For this review, take the finished solid that the model builds, in its own axes (mm). Face numbers are marked on the shaded views. A direction names the side the tool comes from. Give positions to 0.01 mm unless a question says otherwise; leave off trailing zeros. Order: outer loops, then holes, each group sorted by start corner. A loop starts at its lowest first (then second) coordinate and runs counter-clockwise, first axis right, second up. Notation, with made-up numbers: (21.25, 84) - (62.25, 84) arc R5 cw to (62.25, 90) - close; hole circle Ø5 at (21.5, 60.25). An arc over 180 degrees is marked (long way). Put each result on its own line as item: value. Start each with the question number.
```python
from build123d import *

# Parameters (mm, degrees)
SKETCH2_W                                           = 25
SKETCH2_H                                           = 25
BOSS_EXTRUDE1_DEPTH                                 = 10
SKETCH3_W                                           = 20
SKETCH3_H                                           = 20
CUT_EXTRUDE1_DEPTH                                  = 21.310096012
SKETCH5_W                                           = 10
SKETCH5_H                                           = 20
BOSS_EXTRUDE2_DEPTH                                 = 15
SKETCH7_W                                           = 12
SKETCH7_H                                           = 10
CUT_EXTRUDE2_DEPTH                                  = 40.477841886
SKETCH8_R                                           = 2.25
CUT_EXTRUDE3_DEPTH                                  = 49.757050772
SKETCH9_R                                           = 1.75
CUT_EXTRUDE4_DEPTH                                  = 15
SKETCH10_R                                          = 1.75
CUT_EXTRUDE5_DEPTH                                  = 15
CBORE_FOR_M4_HEX_SOCKET_HEAD_CAP_SCREW1_D           = 4.5
CBORE_FOR_M4_HEX_SOCKET_HEAD_CAP_SCREW1_CBORE_D     = 8
CBORE_FOR_M4_HEX_SOCKET_HEAD_CAP_SCREW1_CBORE_DEPTH = 3
CUT_EXTRUDE6_DEPTH                                  = 3


with BuildPart() as part:
    # Sketch2 → Boss-Extrude1 (new body)
    with BuildSketch(Plane.XY):
        Rectangle(SKETCH2_W, SKETCH2_H)
    extrude(amount=BOSS_EXTRUDE1_DEPTH)

    # Sketch3 → Cut-Extrude1 (cut, through all)
    with BuildSketch(Plane.XY.offset(10)):
        with Locations((-2.5, -2.5)):
            Rectangle(SKETCH3_W, SKETCH3_H)
    extrude(amount=-CUT_EXTRUDE1_DEPTH, mode=Mode.SUBTRACT)

    # Sketch5 → Boss-Extrude2 (add)
    with BuildSketch(Plane(origin=(12.5, 0, 0), x_dir=(0, 0, -1), z_dir=(1, 0, 0))):
        with Locations((-5, 16.5)):
            Rectangle(SKETCH5_W, SKETCH5_H)
    extrude(amount=BOSS_EXTRUDE2_DEPTH)

    # Sketch7 → Cut-Extrude2 (cut, through all)
    with BuildSketch(Plane.XY.offset(10)):
        with Locations((21.5, 16.5)):
            Rectangle(SKETCH7_W, SKETCH7_H)
    extrude(amount=-CUT_EXTRUDE2_DEPTH, mode=Mode.SUBTRACT)

    # Sketch8 → Cut-Extrude3 (cut, through all)
    with BuildSketch(Plane(origin=(0, 26.5, 0), x_dir=(1, 0, 0), z_dir=(0, 1, 0))):
        with Locations(Location((22.5, -5, 0), (0, 0, 270))):
            Circle(SKETCH8_R)
    extrude(amount=-CUT_EXTRUDE3_DEPTH, mode=Mode.SUBTRACT)

    # Sketch9 → Cut-Extrude4 (cut)
    with BuildSketch(Plane(origin=(0, 12.5, 0), x_dir=(1, 0, 0), z_dir=(0, 1, 0))):
        with Locations(Location((-2.5, -5, 0), (0, 0, 270))):
            Circle(SKETCH9_R)
    extrude(amount=-CUT_EXTRUDE4_DEPTH, mode=Mode.SUBTRACT)

    # Sketch10 → Cut-Extrude5 (cut)
    with BuildSketch(Plane(origin=(12.5, 0, 0), x_dir=(0, 0, -1), z_dir=(1, 0, 0))):
        with Locations((-5, -2.5)):
            Circle(SKETCH10_R)
    extrude(amount=-CUT_EXTRUDE5_DEPTH, mode=Mode.SUBTRACT)

    # CBORE for M4 Hex Socket Head Cap Screw1 (through all)
    with Locations(Plane(origin=(0, 26.5, 0), x_dir=(1, 0, 0), z_dir=(0, 1, 0))):
        with Locations((22.5, -5)):
            CounterBoreHole(CBORE_FOR_M4_HEX_SOCKET_HEAD_CAP_SCREW1_D / 2, CBORE_FOR_M4_HEX_SOCKET_HEAD_CAP_SCREW1_CBORE_D / 2, CBORE_FOR_M4_HEX_SOCKET_HEAD_CAP_SCREW1_CBORE_DEPTH)

    # Sketch13 → Cut-Extrude6 (cut)
    with BuildSketch(Plane.XZ.offset(-6.5)):
        Polygon((17.881197846, 5), (20.190598923, 1), (24.809401077, 1), (27.118802154, 5), (24.809401077, 9), (20.190598923, 9), align=None)
    extrude(amount=-CUT_EXTRUDE6_DEPTH, mode=Mode.SUBTRACT)


solid = part.part
```
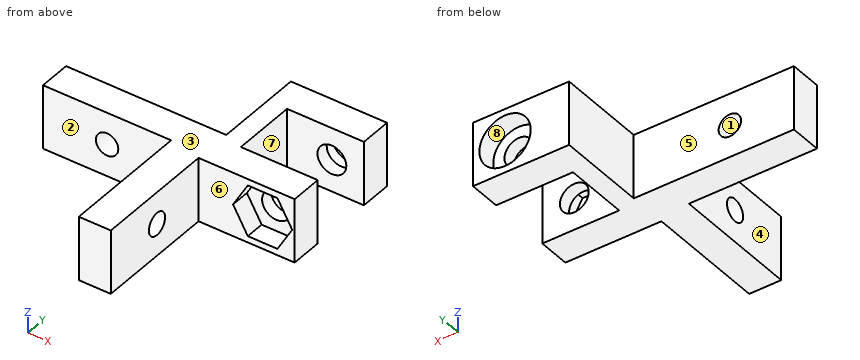
1. Add section B-B, the plane y = 10.5. Give the boundary of the cut face in (x, z).
2. The part is to be moulded in two halves that separate along Z. For the marked faces 1, 2 and 3, say which applies: released by +Z, released by -Z, zero draft, split by the parting line, or undercut.
3. Wall thickness on line 1 (Z direction, x = 22.5, y = 10.55); line 2 (X direction, y = 22.05, z = 5); line 3 (Y direction, x = 21.5, z = 2.75): over which ranges is each line inside the solid? List them lowest first. Write a range as from..to.
4. Add section A-A, the plane x = 17. Give the boundary of the cut face in (y, z).
5. Tool access review of the marked faces 4, 5, 6, 7 and 8: name each direction out of +Z, -Z, +X, -X, +Y, -Y from which nothing blocks a thin tool from reaching the whole face with its end or side.
6. Add section D-D, the plane y = 24. Give the boundary of the cut face in (x, z).
7. Add section C-C, the plane x = 22.5. Give the boundary of the cut face in (y, z), then the cut area to 3 significant figures.
8. Clearance check with flat-ended pins moving along their axes: pin 1 (3 mm diameter, centred on x = -3.5, z = 3, fed in from +Y); pin 2 (3 mm diameter, centred on y = -4, z = 3, fed in from -X); pin 3 (5 mm diameter, centred on y = -6, z = 5, fed in from +X); pin 4 (2 mm diameter, centred on x = -2.5, z = 5, fed in from +Y). State where each tip first meets the part, or that it passes through.
Found:
1. outline: (-12.5, 0) - (27.5, 0) - (27.5, 10) - (-12.5, 10) - close; hole circle Ø3.5 at (-2.5, 5); hole circle Ø4.5 at (22.5, 5)
2. face 1: undercut
2. face 2: zero draft
2. face 3: released by +Z
3. line 1: z = 0..2.75, 7.25..10
3. line 2: x = 12.5..20.25, 24.75..27.5
3. line 3: y = 9.5..11.5, 21.5..23.5
4. outline: (6.5, 0) - (11.5, 0) - (11.5, 10) - (6.5, 10) - close; (21.5, 0) - (26.5, 0) - (26.5, 10) - (21.5, 10) - close
5. face 4: +Z, -Z, -X, -Y
5. face 5: +Z, -Z, -X, +Y
5. face 6: +Z, -Z, +X, -Y
5. face 7: +Z, -Z, +X
5. face 8: +Y
6. outline: (12.5, 0) - (27.5, 0) - (27.5, 10) - (12.5, 10) - close; hole circle Ø8 at (22.5, 5)
7. outline: (6.5, 0) - (11.5, 0) - (11.5, 2.75) - (9.5, 2.75) - (9.5, 1) - (6.5, 1) - close; (6.5, 9) - (9.5, 9) - (9.5, 7.25) - (11.5, 7.25) - (11.5, 10) - (6.5, 10) - close; (21.5, 0) - (26.5, 0) - (26.5, 1) - (23.5, 1) - (23.5, 2.75) - (21.5, 2.75) - close; (21.5, 7.25) - (23.5, 7.25) - (23.5, 9) - (26.5, 9) - (26.5, 10) - (21.5, 10) - close
7. area: 34.0 mm^2
8. pin 1: stops at y = 12.5
8. pin 2: stops at x = 7.5
8. pin 3: stops at x = 12.5
8. pin 4: passes through
